from build123d import *

# Parameters (mm, degrees)
F0_W          = 50.5
F0_H          = 50.5
F1_DEPTH      = 23.7
F2_W          = 45.2
F2_H          = 45.2
F3_DEPTH      = 5
F4_W          = 42
F4_H          = 42
F5_DEPTH      = 5
F5_DEPTH_BACK = 19.5
F6_R          = 2.5
F7_R          = 2
F8_SIZE       = 1
F9_R          = 1


with BuildPart() as f1:
    # F0 (on Top) → F1 (new body)
    with BuildSketch(Plane.XY):
        Rectangle(F0_W, F0_H)
    extrude(amount=F1_DEPTH)

    # F2 (on face) → F3 (join)
    with BuildSketch(Plane.XY.offset(23.7)):
        Rectangle(F2_W, F2_H)
    extrude(amount=F3_DEPTH)

    # F4 (on face) → F5 (cut, two sides)
    with BuildSketch(Plane.XY.offset(23.7)) as f5_sk:
        Rectangle(F4_W, F4_H)
    extrude(amount=F5_DEPTH, mode=Mode.SUBTRACT)
    extrude(f5_sk.sketch, amount=-F5_DEPTH_BACK, mode=Mode.SUBTRACT)

    # F6
    f6_edges = [f1.edges().sort_by_distance(p)[0] for p in [
        (-25.25, 25.25, 11.85),
        (-25.25, -25.25, 11.85),
        (25.25, -25.25, 11.85),
        (25.25, 25.25, 11.85),
        (-22.6, 22.6, 26.2),
        (-22.6, -22.6, 26.2),
        (22.6, -22.6, 26.2),
        (22.6, 22.6, 26.2),
    ]]
    fillet(f6_edges, radius=F6_R)

    # F7
    f7_edges = [f1.edges().sort_by_distance(p)[0] for p in [
        (-21, 21, 16.45),
        (21, 21, 16.45),
        (21, -21, 16.45),
        (-21, -21, 16.45),
    ]]
    fillet(f7_edges, radius=F7_R)

    # F8
    f8_edges = [f1.edges().sort_by_distance(p)[0] for p in [
        (-22.6, 0, 28.7),
    ]]
    chamfer(f8_edges, length=F8_SIZE)

    # F9
    f9_edges = [f1.edges().sort_by_distance(p)[0] for p in [
        (0, 25.25, 0),
    ]]
    fillet(f9_edges, radius=F9_R)


solid = f1.part
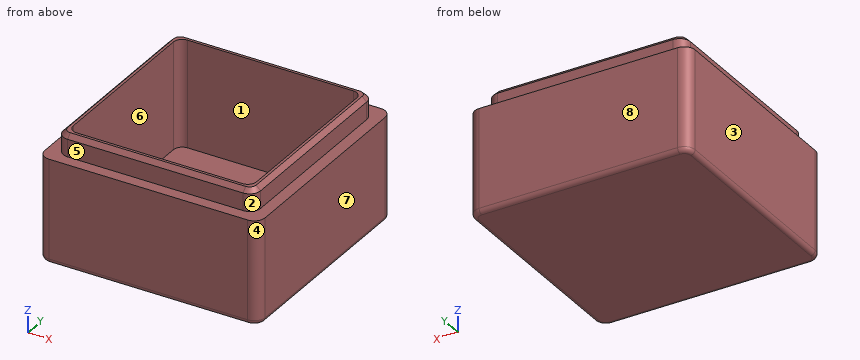
Can you work these out from the model? Positions are in its coordinate system, mm. Face numbers are marked on the shaded views. A direction names the side the tool comes from. Coordinates: 2 decimals unless noted, no trailing zeros. Write each loop counter-clockwise with the first axis right and the second up, starting at its lowest first coordinate (ties: lowest second). Pieces come first, ordered by that corner, then holes. Notation, with made-up numbers: (55.25, 41.5) -> (79.25, 41.5) arc R28 ccw to (79.25, 76.5) -> close; hole circle Ø6 at (-4.5, 86.25). An arc over 180 degrees is marked (long way). Answer as CSV lines item,"result".
1) If we mould it in two halves opening along X, with no side actions, what happens to the marked faces 6, 7 and 8? For each: +X half, -X half, draft (parallel to the pull), parting line (faces both ways), or undercut.
Check result:
face 6,"undercut"
face 7,"+X half"
face 8,"draft"
2) If I drill on line 1 (Y direction, x = -11.5, z = 19.75); line 2 (Y direction, x = -6.5, z = 26), over which ranges is the centre line in solid material (lowest first)? Write a range as from..to.
Check result:
line 1,"-25.25..-21, 21..25.25"
line 2,"-22.6..-21, 21..22.6"
3) Will these pins go through, and if not, where does the flat tip stop? P1, Ø1.2, axis at x = -8, z = 25.5, coming from the +Y side; P2, Ø5, axis at x = 14.5, y = -14.5, coming from the +Z side; P3, Ø3, axis at y = -4.5, z = 26.5, coming from the +X side; P4, Ø3, axis at x = -10, z = 25, coming from the -Y side.
Check result:
P1,"y = 22.6"
P2,"z = 4.2"
P3,"x = 22.6"
P4,"y = -25.25"
4) If we section it at B-B on y = 13.5: Please give me the cut outline in (x, z).
Check result:
outline,"(-25.25, 1) arc R1 ccw to (-24.25, 0) -> (24.25, 0) arc R1 ccw to (25.25, 1) -> (25.25, 23.7) -> (22.6, 23.7) -> (22.6, 27.7) -> (21.6, 28.7) -> (21, 28.7) -> (21, 4.2) -> (-21, 4.2) -> (-21, 28.7) -> (-21.6, 28.7) -> (-22.6, 27.7) -> (-22.6, 23.7) -> (-25.25, 23.7) -> close"
5) On a 3-axis mill with a long thin cutter (end or side, diameter ignored), from which of +Z, -Z, +X, -X, +Y, -Y can I reach the whole of each face in a straight line? I mean the marked faces 1, 2, 3, 4 and 5. Say none if no direction works.
Check result:
face 1,"+Z"
face 2,"+Z, +X, -Y"
face 3,"+Z, -Z, -X, +Y, -Y"
face 4,"+Z, -Z, +X, -Y"
face 5,"+Z, +X, -X, -Y"
6) If we section it at A-A on z = 13.75: Please give me the cut outline in (x, y).
Check result:
outline,"(-25.25, -22.75) arc R2.5 ccw to (-22.75, -25.25) -> (22.75, -25.25) arc R2.5 ccw to (25.25, -22.75) -> (25.25, 22.75) arc R2.5 ccw to (22.75, 25.25) -> (-22.75, 25.25) arc R2.5 ccw to (-25.25, 22.75) -> close; hole (-21, -19) arc R2 ccw to (-19, -21) -> (19, -21) arc R2 ccw to (21, -19) -> (21, 19) arc R2 ccw to (19, 21) -> (-19, 21) arc R2 ccw to (-21, 19) -> close"
